Source: CAD feature listing. Evaluate the final solid. Frame: model axes, mm. Face numbers are marked on the shaded views. A direction names the side the tool comes from. Coordinates: 2 decimals unless noted, no trailing zeros. Loops run counter-clockwise (first coordinate to the right, second up) from the corner with the lowest first, then second, coordinate; pieces in that order, holes last.
```python
from build123d import *

# Parameters (mm, degrees)
SKETCH1_W           = 20
SKETCH1_H           = 50
BOSS_EXTRUDE1_DEPTH = 12
CUT_EXTRUDE1_REACH  = 54.383
SKETCH3_R           = 5
CUT_EXTRUDE3_DEPTH  = 7
CUT_EXTRUDE4_REACH  = 30.553
SKETCH4_R           = 2.25


with BuildPart() as part:
    # Sketch1 → Boss-Extrude1 (new body)
    with BuildSketch(Plane(origin=(0, 0, 0), x_dir=(1, 0, 0), z_dir=(0, 1, 0))):
        Rectangle(SKETCH1_W, SKETCH1_H)
    extrude(amount=BOSS_EXTRUDE1_DEPTH)

    # Sketch2 → Cut-Extrude1 (cut, up to next)
    with BuildSketch(Plane.XY.offset(25), mode=Mode.PRIVATE) as cut_extrude1_sk1:
        Polygon((0, 9.5), (7.25, 9.5), (6.25, 12), (0, 12), (-6.25, 12), (-7.25, 9.5), align=None)
    cut_extrude1_tool1 = extrude(cut_extrude1_sk1.sketch, amount=-CUT_EXTRUDE1_REACH, mode=Mode.PRIVATE) & part.part
    add(cut_extrude1_tool1.solids().sort_by_distance((0, 10.719136, 25))[0], mode=Mode.SUBTRACT)

    # Sketch3 → Cut-Extrude3 (cut)
    with BuildSketch(Plane(origin=(0, 9.5, 0), x_dir=(1, 0, 0), z_dir=(0, 1, 0))):
        with Locations(Location((0, 12.5, 0), (0, 0, 270))):
            Circle(SKETCH3_R)
        with Locations(Location((0, -12.5, 0), (0, 0, 270))):
            Circle(SKETCH3_R)
    extrude(amount=-CUT_EXTRUDE3_DEPTH, mode=Mode.SUBTRACT)

    # Sketch4 → Cut-Extrude4 (cut, up to next)
    with BuildSketch(Plane(origin=(0, 2.5, 0), x_dir=(1, 0, 0), z_dir=(0, 1, 0)), mode=Mode.PRIVATE) as cut_extrude4_sk1:
        with Locations(Location((0, 12.5, 0), (0, 0, 270))):
            Circle(SKETCH4_R)
    cut_extrude4_tool1 = extrude(cut_extrude4_sk1.sketch, amount=-CUT_EXTRUDE4_REACH, mode=Mode.PRIVATE) & part.part
    # Sketch4 → Cut-Extrude4 (cut, up to next)
    with BuildSketch(Plane(origin=(0, 2.5, 0), x_dir=(1, 0, 0), z_dir=(0, 1, 0)), mode=Mode.PRIVATE) as cut_extrude4_sk2:
        with Locations(Location((0, -12.5, 0), (0, 0, 270))):
            Circle(SKETCH4_R)
    cut_extrude4_tool2 = extrude(cut_extrude4_sk2.sketch, amount=-CUT_EXTRUDE4_REACH, mode=Mode.PRIVATE) & part.part
    add(cut_extrude4_tool1.solids().sort_by_distance((0, 2.5, -12.5))[0], mode=Mode.SUBTRACT)
    add(cut_extrude4_tool2.solids().sort_by_distance((0, 2.5, 12.5))[0], mode=Mode.SUBTRACT)


solid = part.part
```
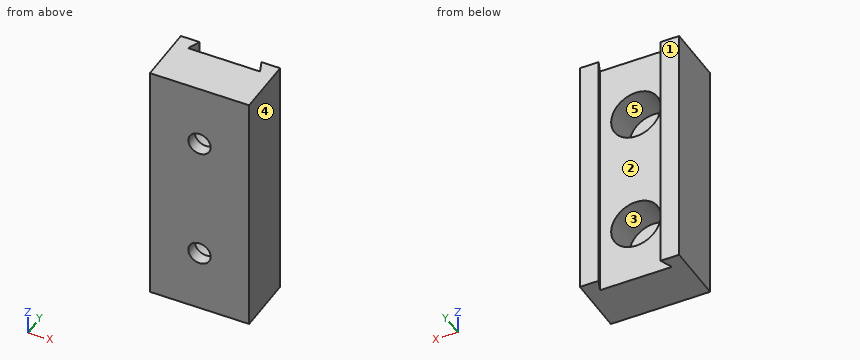
Q1. Section query C-C on y = 6.5. Return the cut outline in (x, z), then the cut area to 3 significant figures.
Q2. Section query D-D on z = 2.5. Return the cut outline in (x, y).
Q3. Reachability of the marked faces 4 and 5 from +Z, -Z, +X, -X, +Y, -Y: full face, straight path, thin tool, end or side. Return the list, or none.
Q4. Section query A-A on z = 12.5. Return the cut outline in (x, y), then the cut area to 3 significant figures.
Q5. Section query B-B on x = 0. Return the cut outline in (y, z), then the cut area to 4 significant figures.
Q6. Draft query along Y for the marked faces 1, 2 and 3. Return one class per face: released by +Y, released by -Y, zero draft, split by the parting line, or undercut.
Q7. Material intervals for line 1 along X through (y, z) = (7.5, -12.5); line 2 along X through (y, z) = (1.4, -12.5); line 3 along Z through (x, y) = (-1, 8.25), sorted ascending.
Q8. First-contact query: pin 1 Ø3 at (x, z) = (0.5, -13) entering from +Y; pin 2 Ø11.5 at (x, z) = (-1.5, -5.5) entering from +Y; pin 3 Ø1.5 at (x, z) = (2.5, 6) entering from +Y. Flat tips, straight axial feed; report the tip coordinate or a pass-through.
Resolved:
1. outline: (-10, -25) - (10, -25) - (10, 25) - (-10, 25) - close; hole circle Ø10 at (0, -12.5); hole circle Ø10 at (0, 12.5)
1. area: 843 mm2
2. outline: (-10, 0) - (10, 0) - (10, 12) - (6.25, 12) - (7.25, 9.5) - (-7.25, 9.5) - (-6.25, 12) - (-10, 12) - close
3. face 4: +Z, -Z, +X, +Y, -Y
3. face 5: +Y
4. outline: (-10, 0) - (-2.25, 0) - (-2.25, 2.5) - (-5, 2.5) - (-5, 9.5) - (-7.25, 9.5) - (-6.25, 12) - (-10, 12) - close; (2.25, 0) - (10, 0) - (10, 12) - (6.25, 12) - (7.25, 9.5) - (5, 9.5) - (5, 2.5) - (2.25, 2.5) - close
4. area: 125 mm2
5. outline: (0, -25) - (9.5, -25) - (9.5, -17.5) - (2.5, -17.5) - (2.5, -14.75) - (0, -14.75) - close; (0, -10.25) - (2.5, -10.25) - (2.5, -7.5) - (9.5, -7.5) - (9.5, 7.5) - (2.5, 7.5) - (2.5, 10.25) - (0, 10.25) - close; (0, 14.75) - (2.5, 14.75) - (2.5, 17.5) - (9.5, 17.5) - (9.5, 25) - (0, 25) - close
5. area: 312.5 mm2
6. face 1: released by +Y
6. face 2: undercut
6. face 3: zero draft
7. line 1: x = -10 to -5, 5 to 10
7. line 2: x = -10 to -2.25, 2.25 to 10
7. line 3: z = -25 to -17.4, -7.6 to 7.6, 17.4 to 25
8. pin 1: passes through
8. pin 2: stops at y = 12
8. pin 3: stops at y = 9.5
